Verification items for the finished model (mm, model axes). A direction names the side the tool comes from. Coordinates: 2 decimals unless noted, no trailing zeros. Order: outer loops, then holes, each group sorted by start corner. A loop starts at its lowest first (then second) coordinate and runs counter-clockwise, first axis right, second up. Notation, with made-up numbers: M 24,-38 L 62,-38 A34 ccw 62,-5 Z; hole C -12,8.5 d9. An arc over 180 degrees is marked long. Return JSON: item names as keys, results as strings.
```python
from build123d import *

# Parameters (mm, degrees)
F1_DEPTH = 60.325
F3_D     = 50.8
F5_DEPTH = 88.901


with BuildPart() as f1:
    # F0 (on Front) → F1 (new body)
    with BuildSketch(Plane.XZ):
        Polygon((0, 88.9), (0, 0), (19.05, 0), (57.15, 25.4), (101.6, 25.4), (107.95, 19.05), (187.325, 19.05), (187.325, 88.9), align=None)
    extrude(amount=F1_DEPTH)

    # F3 (through all)
    with Locations(Plane.XY.offset(88.9)):
        with Locations((152.4, -30.1625)):
            Hole(F3_D / 2)

    # F4 (on face) → F5 (cut, through all)
    with BuildSketch(Plane.XY.offset(88.9)):
        Polygon((9.525, -9.525), (0, -15.024261), (0, -46.888239), (9.525, -52.3875), align=None)
    extrude(amount=-F5_DEPTH, mode=Mode.SUBTRACT)


solid = f1.part
```
Q1. Tool access check on faces 1 (the face through (129, -43, 19.05)), 2 (the face through (37.8, -29.7, 12.5)), 3 (the face through (9.525, -31, 45)). Record the directions out of +Z, -Z, +X, -X, +Y, -Y that give a thin tool (end or side, any length) a straight path to the whole face; none if there is none.
Values:
{"face 1": "-Z, +X, +Y, -Y", "face 2": "-Z, +Y, -Y", "face 3": "+Z, -Z"}
Q2. Material ranges on line 1 along Y through (x, z) = (152, 47) (3 decimals); line 2 along Z through (x, y) = (64, -6); line 3 along X through (y, z) = (-29.5, 74) (3 decimals), recorded low to high.
Values:
{"line 1": "-60.325 to -55.559, -4.766 to 0", "line 2": "25.4 to 88.9", "line 3": "9.525 to 127.009, 177.791 to 187.325"}
Q3. Cross-section at B-B, the plane y = -18.5. Record the boundary of the cut face in (x, z) (3 decimals).
Values:
{"outline": "M 9.525,0 L 19.05,0 L 57.15,25.4 L 101.6,25.4 L 107.95,19.05 L 129.836,19.05 L 129.836,88.9 L 9.525,88.9 Z; M 174.964,19.05 L 187.325,19.05 L 187.325,88.9 L 174.964,88.9 Z"}
Q4. Cross-section at D-D, the plane z = 47.5. Record the boundary of the cut face in (x, y) (1 decimal), and give its area (3 significant figures).
Values:
{"outline": "M 0,-60.3 L 187.3,-60.3 L 187.3,0 L 0,0 L 0,-15 L 9.5,-9.5 L 9.5,-52.4 L 0,-46.9 Z; hole C 152.4,-30.2 d50.8", "area": "8,920 mm^2"}
Q5. Draft check along Y on faces 4 (the face through (95, -30, 88.9)), 5 (the face through (92, 0, 55)), 6 (the face through (4.7, -49.6, 45.1)). Enter one of: pulls with the +Y half, pulls with the -Y half, needs draft (parallel to the pull), parting line crosses it, or undercut.
Values:
{"face 4": "needs draft", "face 5": "pulls with the +Y half", "face 6": "undercut"}
Q6. Cross-section at C-C, the plane z = 21.5. Record the boundary of the cut face in (x, y) (1 decimal), and give its area (3 significant figures).
Values:
{"outline": "M 0,-60.3 L 51.3,-60.3 L 51.3,0 L 0,0 L 0,-15 L 9.5,-9.5 L 9.5,-52.4 L 0,-46.9 Z; M 105.5,-60.3 L 187.3,-60.3 L 187.3,0 L 105.5,0 Z; hole C 152.4,-30.2 d50.8", "area": "5,650 mm^2"}
Q7. Go/stop test with flat-tipped pins: pin 1 (21.5 mm diameter, centred on y = -28, z = 43, fed in from -X) (3 decimals); pin 2 (10 mm diameter, centred on x = 111.5, y = -16, fed in from -Z); pin 3 (6 mm diameter, centred on y = -44.5, z = 52.5, fed in from -X); pin 4 (2 mm diameter, centred on y = -26, z = 11.5, fed in from +X). Record where each tip stops, or that it passes through.
Values:
{"pin 1": "x = 9.525", "pin 2": "z = 19.05", "pin 3": "x = 0", "pin 4": "x = 37.8"}
